Input: part model. Units: mm. Frame: model coordinates. A direction names the side the tool comes from. Round coordinates to 2 decimals unless told otherwise and drop trailing zeros. Write each loop counter-clockwise with the first axis right and the second up, starting at its lowest first coordinate (ties: lowest second). Pieces come first, ordered by that corner, then holes. Notation, with made-up numbers: (63.5, -16.5) -> (118.5, -16.5) arc R18 ccw to (118.5, -8.5) -> close; hole circle Ø4 at (4, -1). An arc over 180 degrees is marked (long way). Write item = value, one per line. Start each with the question number.
```python
from build123d import *

# Parameters (mm, degrees)
RESSALTO_EXTRUS_O1_DEPTH        = 2
ESBO_O2_R                       = 1.5
CORTE_EXTRUS_O1_DEPTH           = 3
CORTE_EXTRUS_O1_TAPER           = -40
ESPELHAR3_COPY_1_SKETCH_R       = 1.5
ESPELHAR3_COPY_1_DEPTH          = 3
ESPELHAR3_COPY_1_TAPER          = -40
PADR_OCIRCULAR1_COUNT           = 2
PADR_OCIRCULAR1_ANGLE           = 90
PADR_OCIRCULAR1_COPY_1_SKETCH_R = 1.5
PADR_OCIRCULAR1_COPY_1_DEPTH    = 3
PADR_OCIRCULAR1_COPY_1_TAPER    = -40
PADR_OCIRCULAR1_COPY_2_SKETCH_R = 1.5
PADR_OCIRCULAR1_COPY_2_DEPTH    = 3
PADR_OCIRCULAR1_COPY_2_TAPER    = -40
PADR_OCIRCULAR1_COPY_3_SKETCH_R = 1.5
PADR_OCIRCULAR1_COPY_3_DEPTH    = 3
PADR_OCIRCULAR1_COPY_3_TAPER    = -40


with BuildPart() as part:
    # Esboço1 → Ressalto-extrusão1 (new body)
    with BuildSketch(Plane(origin=(0, 0, 0), x_dir=(1, 0, 0), z_dir=(0, 1, 0))):
        Polygon((-20, 35), (-20, 45), (0, 45), (0, 29.131440421), (-6, 29.131440421), (-6, 14.131440421), (0, 14.131440421), (0, -13.868559579), (-6, -13.868559579), (-6, -28.868559579), (0, -28.868559579), (0, -45), (-20, -45), (-20, -35), (-35, -20), (-45, -20), (-45, 20), (-35, 20), align=None)
        with BuildLine():
            Line((-27, -5.868559579), (-6, -5.868559579))
            ThreePointArc((-6, -5.868559579), (-4.585786438, -5.282773141), (-4, -3.868559579))
            Line((-4, -3.868559579), (-4, 4.131440421))
            ThreePointArc((-4, 4.131440421), (-4.585786438, 5.545653984), (-6, 6.131440421))
            Line((-6, 6.131440421), (-27, 6.131440421))
            ThreePointArc((-27, 6.131440421), (-28.414213562, 5.545653984), (-29, 4.131440421))
            Line((-29, 4.131440421), (-29, -3.868559579))
            ThreePointArc((-29, -3.868559579), (-28.414213562, -5.282773141), (-27, -5.868559579))
        make_face(mode=Mode.SUBTRACT)
    ressalto_extrus_o1 = extrude(amount=RESSALTO_EXTRUS_O1_DEPTH)

    # Espelhar1: Ressalto-extrusão1 across plane
    add(ressalto_extrus_o1.mirror(Plane(origin=(0, 0, 0), x_dir=(0, 0, 1), z_dir=(1, 0, 0))))

    # Esboço2 → Corte-extrusão1 (cut, through all)
    with BuildSketch(Plane(origin=(0, 2, 0), x_dir=(1, 0, 0), z_dir=(0, 1, 0))):
        with Locations((-15, 37)):
            Circle(ESBO_O2_R)
    corte_extrus_o1 = extrude(amount=-CORTE_EXTRUS_O1_DEPTH, taper=CORTE_EXTRUS_O1_TAPER, mode=Mode.SUBTRACT)

    # Espelhar2: Corte-extrusão1 across plane
    add(corte_extrus_o1.mirror(Plane(origin=(0, 0, 0), x_dir=(0, 0, 1), z_dir=(1, 0, 0))), mode=Mode.SUBTRACT)

    # Espelhar3: Corte-extrusão1 across plane
    add(corte_extrus_o1.mirror(Plane.XY), mode=Mode.SUBTRACT)

    # Espelhar3 copy 1 sketch → Espelhar3 copy 1 (cut, through all)
    with BuildSketch(Plane(origin=(0, 2, 0), x_dir=(-1, 0, 0), z_dir=(0, 1, 0))):
        with Locations((-15, 37)):
            Circle(ESPELHAR3_COPY_1_SKETCH_R)
    extrude(amount=-ESPELHAR3_COPY_1_DEPTH, taper=ESPELHAR3_COPY_1_TAPER, mode=Mode.SUBTRACT)

    # PadrãoCircular1: Corte-extrusão1 ×2 about axis
    padr_ocircular1_axis = Axis((0, 0, 0), (0, -1, 0))
    for i in range(1, PADR_OCIRCULAR1_COUNT):
        add(corte_extrus_o1.rotate(padr_ocircular1_axis, i * PADR_OCIRCULAR1_ANGLE / (PADR_OCIRCULAR1_COUNT - 1)), mode=Mode.SUBTRACT)

    # PadrãoCircular1 copy 1 sketch → PadrãoCircular1 copy 1 (cut, through all)
    with BuildSketch(Plane.ZX.offset(2)):
        with Locations((-15, -37)):
            Circle(PADR_OCIRCULAR1_COPY_1_SKETCH_R)
    extrude(amount=-PADR_OCIRCULAR1_COPY_1_DEPTH, taper=PADR_OCIRCULAR1_COPY_1_TAPER, mode=Mode.SUBTRACT)

    # PadrãoCircular1 copy 2 sketch → PadrãoCircular1 copy 2 (cut, through all)
    with BuildSketch(Plane(origin=(0, 2, 0), x_dir=(0, 0, -1), z_dir=(0, 1, 0))):
        with Locations((-15, 37)):
            Circle(PADR_OCIRCULAR1_COPY_2_SKETCH_R)
    extrude(amount=-PADR_OCIRCULAR1_COPY_2_DEPTH, taper=PADR_OCIRCULAR1_COPY_2_TAPER, mode=Mode.SUBTRACT)

    # PadrãoCircular1 copy 3 sketch → PadrãoCircular1 copy 3 (cut, through all)
    with BuildSketch(Plane(origin=(0, 2, 0), x_dir=(0, 0, -1), z_dir=(0, 1, 0))):
        with Locations((-15, -37)):
            Circle(PADR_OCIRCULAR1_COPY_3_SKETCH_R)
    extrude(amount=-PADR_OCIRCULAR1_COPY_3_DEPTH, taper=PADR_OCIRCULAR1_COPY_3_TAPER, mode=Mode.SUBTRACT)


solid = part.part
```
1. Pin query (flat end, axial travel): P1, Ø1, axis at y = 1, z = 24, coming from the +X side; P2, Ø0.6, axis at y = 1.5, z = -41.5, coming from the +X side; P3, Ø0.6, axis at y = 1, z = 24, coming from the -X side; P4, Ø12, axis at x = -28, z = 31, coming from the -Y side. Return the tip coordinate at first contact, or that it passes through.
2. Section D-D (x = -37). State how many separate pieces and enclosed holes the cut face has, then the cut area to 3 significant figures.
3. Section B-B (z = 23.5). Output: boundary loops of the cut face in (x, y).
4. Section A-A (x = -15). Output: boundary loops of the cut face in (y, z), then the cut area to 3 significant figures.
5. Line query: line 1 along X through (y, z) = (0.3, 28); line 2 along X through (y, z) = (0.4, 13); line 3 along X through (y, z) = (0.15, 17). Output: solid intervals per line, ascending.
6. Section C-C (z = 2.5). Output: boundary loops of the cut face in (x, y), then the cut area to 3 significant figures.
7. Reachability of faces 1 (the flat face through (28, 1, -27)), 2 (the flat face through (-20, 1, 40)), 3 (the flat face through (0, 1, -45)), 4 (the flat face through (6, 1, -22)), 5 (the flat face through (20, 1, 40)) from +Z, -Z, +X, -X, +Y, -Y: full face, straight path, thin tool, end or side. Return the list, or none.
8. Mould query, pull axis X, two halves, no side actions, for faces 6 (the cylindrical face through (-4.57, 0.99, -5.53)), 7 (the flat face through (-40, 1, -20)), 8 (the flat face through (-29, 1, 0)), 9 (the flat face through (45, 1, 0)). Classes: pulls with the +X half, pulls with the -X half, needs draft (parallel to the pull), parting line crosses it, or undercut.
Check sheet entries:
q1.P1 = 31.5
q1.P2 = 20
q1.P3 = -31.3
q1.P4 = 0
q2.separate_pieces = 3
q2.enclosed_holes = 0
q2.area = 61.3 mm2
q3.outline = (-31.5, 0) -> (-6, 0) -> (-6, 2) -> (-31.5, 2) -> close; (6, 0) -> (31.5, 0) -> (31.5, 2) -> (6, 2) -> close
q4.outline = (0, -45) -> (2, -45) -> (2, -38.5) -> (0, -40.18) -> close; (0, -33.82) -> (2, -35.5) -> (2, -6.13) -> (0, -6.13) -> close; (0, 5.87) -> (2, 5.87) -> (2, 35.5) -> (0, 33.82) -> close; (0, 40.18) -> (2, 38.5) -> (2, 45) -> (0, 45) -> close
q4.area = 137 mm2
q5.line_1 = -27 to -6, 6 to 27
q5.line_2 = -45 to -39.02, -34.98 to 34.98, 39.02 to 45
q5.line_3 = -45 to -39.31, -34.69 to -6, 6 to 34.69, 39.31 to 45
q6.outline = (-45, 0) -> (-29, 0) -> (-29, 2) -> (-45, 2) -> close; (-4, 0) -> (4, 0) -> (4, 2) -> (-4, 2) -> close; (29, 0) -> (45, 0) -> (45, 2) -> (29, 2) -> close
q6.area = 80.0 mm2
q7.face_1 = -Z, +X, +Y, -Y
q7.face_2 = +Z, -X, +Y, -Y
q7.face_3 = -Z, +X, -X, +Y, -Y
q7.face_4 = +Y, -Y
q7.face_5 = +Z, +X, +Y, -Y
q8.face_6 = undercut
q8.face_7 = needs draft
q8.face_8 = undercut
q8.face_9 = pulls with the +X half
